Autodesk Inventor part; units mm, degrees
ref_plane "YZ Plane" through (0, 0, 0) normal (1, 0, 0) x (0, 1, 0)
ref_plane "XZ Plane" through (0, 0, 0) normal (0, 1, 0) x (-1, 0, 0)
ref_plane "XY Plane" through (0, 0, 0) normal (0, 0, 1) x (1, 0, 0)
sketch "Sketch1" plane through (0, 0, 0) normal (0, 1, 0) x (-1, 0, 0)
  line L0 (53.5, 75) -> (-53.5, 75)
  line L1 (-53.5, 75) -> (-53.5, -75)
  line L2 (-53.5, -75) -> (53.5, -75)
  line L3 (53.5, -75) -> (53.5, 75)
  line L4 (74.9, 0) -> (-74.9, 0)
  line L5 (0, -105) -> (0, 105)
  point P0 (0, 0)
  point P1 (0, 75)
  point P2 (53.5, 0)
  dimension "d0" = 150
  dimension "d1" = 107
extrude "Extrusion1" add sketch "Sketch1" along normal blind 3.175
sketch "Sketch2" plane through (0, 3.175, 0) normal (0, 1, 0) x (1, 0, 0)
  line L0 (-53.5, -75) -> (53.5, -75)
  line L1 (-53.5, 75) -> (-53.5, -75)
  line L2 (53.5, 75) -> (-53.5, 75)
  line L3 (-33.5, -30) -> (33.5, -30)
  line L4 (33.5, -30) -> (33.5, 30) construction
  line L5 (33.5, 30) -> (-33.5, 30) construction
  line L6 (-33.5, 30) -> (-33.5, -30) construction
  line L7 (-74.9, 0) -> (74.9, 0)
  line L8 (0, 105) -> (0, -105)
  line L9 (-17.5, -10.5) -> (17.5, -10.5)
  point P0 (0, -30)
  point P1 (-33.5, 0)
  point P2 (0, -10.5)
  point P3 (0, -7.5)
  point P4 (0, 7.5)
  dimension "d11" = 45
  dimension "d12" = 20
  dimension "d13" = 64.5
  dimension "d14" = 35
  dimension "d15" = 7.5
  dimension "d16" = 7.5
hole "Hole1" at (-17.5, 3.175, 10.5) at (17.5, 3.175, 10.5) at (-33.5, 3.175, 30) at (-33.5, 3.175, -30) at (33.5, 3.175, -30) at (33.5, 3.175, 30) direction (0, -1, 0) diameter 4 end through all
hole "Hole2" at (0, 3.175, 7.5) at (0, 3.175, -7.5) direction (0, -1, 0) diameter 4 end through all
properties part number "base superior"
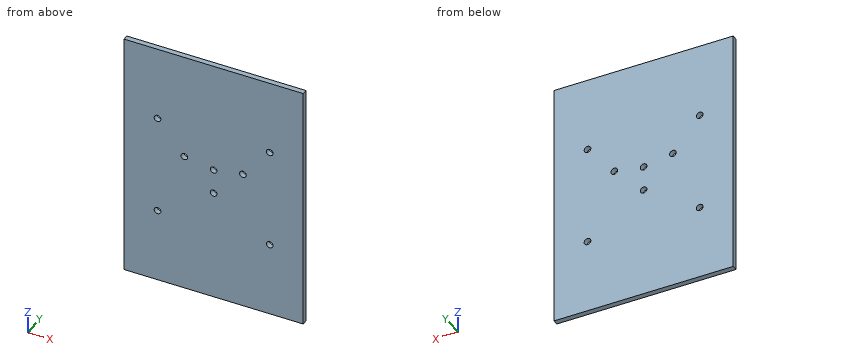
Geometry check sheet. Reference: the model listing, model coordinates, mm. Give positions to 0.01 mm unless a question says otherwise; leave off trailing zeros. Write each loop counter-clockwise with the first axis right and the second up, starting at its lowest first coordinate (ties: lowest second). Pieces come first, ordered by that corner, then holes. Notation, with made-up numbers: (82.5, 72) - (93.5, 72) arc R14 cw to (93.5, 90) - close; hole circle Ø2 at (46, -30.75). An arc over 180 degrees is marked (long way). Use a Markdown table: item, result.
Q1. Thickness scan on L1, parallel to X at y = 1.3, z = 30; L2, parallel to Z at x = 33.5, y = 2.5; L3, parallel to X at y = 1.15, z = 10.5. Record the ranges inside material, lowest first. Write a range as [from, to].
Computed:
| item | result |
|---|---|
| L1 | x = [-53.5, -35.5], [-31.5, 31.5], [35.5, 53.5] |
| L2 | z = [-75, -32], [-28, 28], [32, 75] |
| L3 | x = [-53.5, -19.5], [-15.5, 15.5], [19.5, 53.5] |
Q2. Section check A-A, the plane x = -33.5. Enter the section's corners in (y, z) (3 decimals).
Computed:
| item | result |
|---|---|
| outline | (0, -75) - (3.175, -75) - (3.175, -32) - (0, -32) - close; (0, -28) - (3.175, -28) - (3.175, 28) - (0, 28) - close; (0, 32) - (3.175, 32) - (3.175, 75) - (0, 75) - close |
Q3. Section check D-D, the plane x = 17.5. Enter the section's corners in (y, z) (3 decimals).
Computed:
| item | result |
|---|---|
| outline | (0, -75) - (3.175, -75) - (3.175, 8.5) - (0, 8.5) - close; (0, 12.5) - (3.175, 12.5) - (3.175, 75) - (0, 75) - close |
Q4. Section check C-C, the plane z = -7.5. Enter the section's corners in (x, y) (3 decimals), then the cut area to 3 significant figures.
Computed:
| item | result |
|---|---|
| outline | (-53.5, 0) - (-2, 0) - (-2, 3.175) - (-53.5, 3.175) - close; (2, 0) - (53.5, 0) - (53.5, 3.175) - (2, 3.175) - close |
| area | 327 mm² |
Q5. Section check B-B, the plane z = -30. Enter the section's corners in (x, y) (3 decimals).
Computed:
| item | result |
|---|---|
| outline | (-53.5, 0) - (-35.5, 0) - (-35.5, 3.175) - (-53.5, 3.175) - close; (-31.5, 0) - (31.5, 0) - (31.5, 3.175) - (-31.5, 3.175) - close; (35.5, 0) - (53.5, 0) - (53.5, 3.175) - (35.5, 3.175) - close |
Q6. Go/stop test with a flat-tipped pin: P1, Ø3.5, axis at x = 0, z = -7.5, coming from the -Y side. Record where the tip stops, or that it passes through.
Computed:
| item | result |
|---|---|
| P1 | passes through |
